Geometry check sheet. Reference: the model listing, model coordinates, mm. Coordinates: 2 decimals unless noted, no trailing zeros. Loops run counter-clockwise (first coordinate to the right, second up) from the corner with the lowest first, then second, coordinate; pieces in that order, holes last. Notation, with made-up numbers: (50, 7) -> (59, 7) arc R12 ccw to (59, 18) -> close; hole circle Ø10 at (38, 80). An arc over 180 degrees is marked (long way). Answer as a JSON object with one key per item and string values.
Autodesk Inventor part; units mm, degrees
ref_plane "YZ Plane" through (0, 0, 0) normal (1, 0, 0) x (0, 1, 0)
ref_plane "XZ Plane" through (0, 0, 0) normal (0, 1, 0) x (-1, 0, 0)
ref_plane "XY Plane" through (0, 0, 0) normal (0, 0, 1) x (1, 0, 0)
sketch "スケッチ1" plane through (0, 0, 0) normal (0, 0, 1) x (1, 0, 0)
  arc A0 (-16.2703, -9.5731) -> (-13.6889, -8.0827) centre (-16.2703, -6.5923) ccw
  arc A1 (-16.2703, -9.5731) -> (-17.2313, -10.1279) centre (-16.2703, -10.6827) ccw
  arc A2 (-17.2313, -10.1279) -> (-17.2313, -11.2375) centre (-16.2703, -10.6827) ccw
  arc A3 (-17.2313, -14.2183) -> (-17.2313, -11.2375) centre (-19.8127, -12.7279) ccw
  arc A4 (-17.2313, -14.2183) -> (-17.2313, -15.3279) centre (-16.2703, -14.7731) ccw
  arc A5 (-17.2313, -15.3279) -> (-16.2703, -15.8827) centre (-16.2703, -14.7731) ccw
  arc A6 (-13.6889, -17.3731) -> (-16.2703, -15.8827) centre (-16.2703, -18.8635) ccw
  arc A7 (-13.6889, -17.3731) -> (-12.7279, -17.9279) centre (-12.7279, -16.8183) ccw
  arc A8 (-12.7279, -17.9279) -> (-11.767, -17.3731) centre (-12.7279, -16.8183) ccw
  arc A9 (-9.1855, -15.8827) -> (-11.767, -17.3731) centre (-9.1855, -18.8635) ccw
  arc A10 (-9.1855, -15.8827) -> (-8.2246, -15.3279) centre (-9.1855, -14.7731) ccw
  arc A11 (-8.2246, -15.3279) -> (-8.2246, -14.2183) centre (-9.1855, -14.7731) ccw
  arc A12 (-8.2246, -11.2375) -> (-8.2246, -14.2183) centre (-5.6431, -12.7279) ccw
  arc A13 (-8.2246, -11.2375) -> (-8.2246, -10.1279) centre (-9.1855, -10.6827) ccw
  arc A14 (-8.2246, -10.1279) -> (-9.1855, -9.5731) centre (-9.1855, -10.6827) ccw
  arc A15 (-11.767, -8.0827) -> (-9.1855, -9.5731) centre (-9.1855, -6.5923) ccw
  arc A16 (-11.767, -8.0827) -> (-12.7279, -7.5279) centre (-12.7279, -8.6375) ccw
  arc A17 (-12.7279, -7.5279) -> (-13.6889, -8.0827) centre (-12.7279, -8.6375) ccw
  circle A18 centre (-12.7279, -12.7279) radius 1.5 construction
  circle A19 centre (-12.7279, -12.7279) radius 1.5
  circle A20 centre (-12.7279, -12.7279) radius 6
  point P0 (0, 0)
  point P1 (0, 0)
  dimension "d0" = 3
extrude "押し出し1" add sketch "スケッチ1" along normal blind 5 contours A0 A17 A16 A15 A14 A13 A12 A11 A10 A9 A8 A7 A6 A5 A4 A3 A2 A1
chamfer "面取り1" distance 1 angle 45 1 edges at (-14.2279, -12.7279, 0)
sketch "書きだし" plane through (0, 0, 5) normal (0, 0, 1) x (1, 0, 0)
  arc A0 (-17.2313, -14.2183) -> (-16.2703, -15.8827) centre (-16.2703, -14.7731) ccw
  arc A1 (-13.6889, -17.3731) -> (-16.2703, -15.8827) centre (-16.2703, -18.8635) ccw
  arc A2 (-13.6889, -17.3731) -> (-11.767, -17.3731) centre (-12.7279, -16.8183) ccw
  arc A3 (-9.1855, -15.8827) -> (-11.767, -17.3731) centre (-9.1855, -18.8635) ccw
  arc A4 (-9.1855, -15.8827) -> (-8.2246, -14.2183) centre (-9.1855, -14.7731) ccw
  arc A5 (-8.2246, -11.2375) -> (-8.2246, -14.2183) centre (-5.6431, -12.7279) ccw
  arc A6 (-8.2246, -11.2375) -> (-9.1855, -9.5731) centre (-9.1855, -10.6827) ccw
  arc A7 (-11.767, -8.0827) -> (-9.1855, -9.5731) centre (-9.1855, -6.5923) ccw
  arc A8 (-11.767, -8.0827) -> (-13.6889, -8.0827) centre (-12.7279, -8.6375) ccw
  arc A9 (-16.2703, -9.5731) -> (-13.6889, -8.0827) centre (-16.2703, -6.5923) ccw
  arc A10 (-16.2703, -9.5731) -> (-17.2313, -11.2375) centre (-16.2703, -10.6827) ccw
  arc A11 (-17.2313, -14.2183) -> (-17.2313, -11.2375) centre (-19.8127, -12.7279) ccw
  circle A12 centre (-12.7279, -12.7279) radius 1.5
  point P0 (0, 0)
properties part number "原動節接続部v2内-2" material "アルミニウム 2014-T4"
1. Section check A-A, the plane z = 4.05. Record the boundary of the cut face in (x, y), then the cut area to 3 significant figures.
Evaluation:
{"outline": "(-17.23, -15.33) arc R1.11 ccw to (-16.27, -15.88) arc R2.98 cw to (-13.69, -17.37) arc R1.11 ccw to (-12.73, -17.93) arc R1.11 ccw to (-11.77, -17.37) arc R2.98 cw to (-9.19, -15.88) arc R1.11 ccw to (-8.22, -15.33) arc R1.11 ccw to (-8.22, -14.22) arc R2.98 cw to (-8.22, -11.24) arc R1.11 ccw to (-8.22, -10.13) arc R1.11 ccw to (-9.19, -9.57) arc R2.98 cw to (-11.77, -8.08) arc R1.11 ccw to (-12.73, -7.53) arc R1.11 ccw to (-13.69, -8.08) arc R2.98 cw to (-16.27, -9.57) arc R1.11 ccw to (-17.23, -10.13) arc R1.11 ccw to (-17.23, -11.24) arc R2.98 cw to (-17.23, -14.22) arc R1.11 ccw to start; hole circle Ø3 at (-12.73, -12.73)", "area": "59.7 mm^2"}
2. Section check B-B, the plane y = -16.5. Record the boundary of the cut face in (x, z), then the cut area to 3 significant figures.
Evaluation:
{"outline": "(-14.45, 0) -> (-11, 0) -> (-11, 5) -> (-14.45, 5) -> close", "area": "17.3 mm^2"}
3. Depth check by flat-ended pin: P1, Ø3, axis at x = -10, z = 2.5, coming from the -Y side; P2, Ø1.5, axis at x = -13, z = 3, coming from the +Y side; P3, Ø1.5, axis at y = -9.5, z = 3, coming from the -X side; P4, Ø2, axis at x = -12.5, y = -14, coming from the -Z side. Enter the tip coordinate at first touch or a pass-through.
Evaluation:
{"P1": "stops at y = -16.99", "P2": "stops at y = -7.53", "P3": "stops at x = -17.29", "P4": "stops at z = 0.21"}
4. Thickness scan on probe 1 along X at (y, z) = (-12.75, 3); probe 2 along Y at (x, z) = (-11.75, 2.55); probe 3 along X at (y, z) = (-11.5, 2.5). Record the ranges inside material, lowest first. Write a range as from..to.
Evaluation:
{"probe 1": "x = -16.83..-14.23, -11.23..-8.62", "probe 2": "y = -17.34..-13.87, -11.59..-8.11", "probe 3": "x = -17.1..-13.59, -11.87..-8.36"}
5. Section check C-C, the plane x = -16.5. Record the boundary of the cut face in (y, z).
Evaluation:
{"outline": "(-15.86, 0) -> (-9.6, 0) -> (-9.6, 5) -> (-15.86, 5) -> close"}
6. Mould release check, pull along Y, two halves, no side actions. Record for faces 1 (the face through (-12.18, -7.673, 2.465)), 2 (the face through (-10.69, -16.29, 2.46)), 3 (the face through (-16.83, -12.71, 2.46)): released by +Y, released by -Y, zero draft, split by the parting line, or undercut.
Evaluation:
{"face 1": "released by +Y", "face 2": "released by -Y", "face 3": "undercut"}
